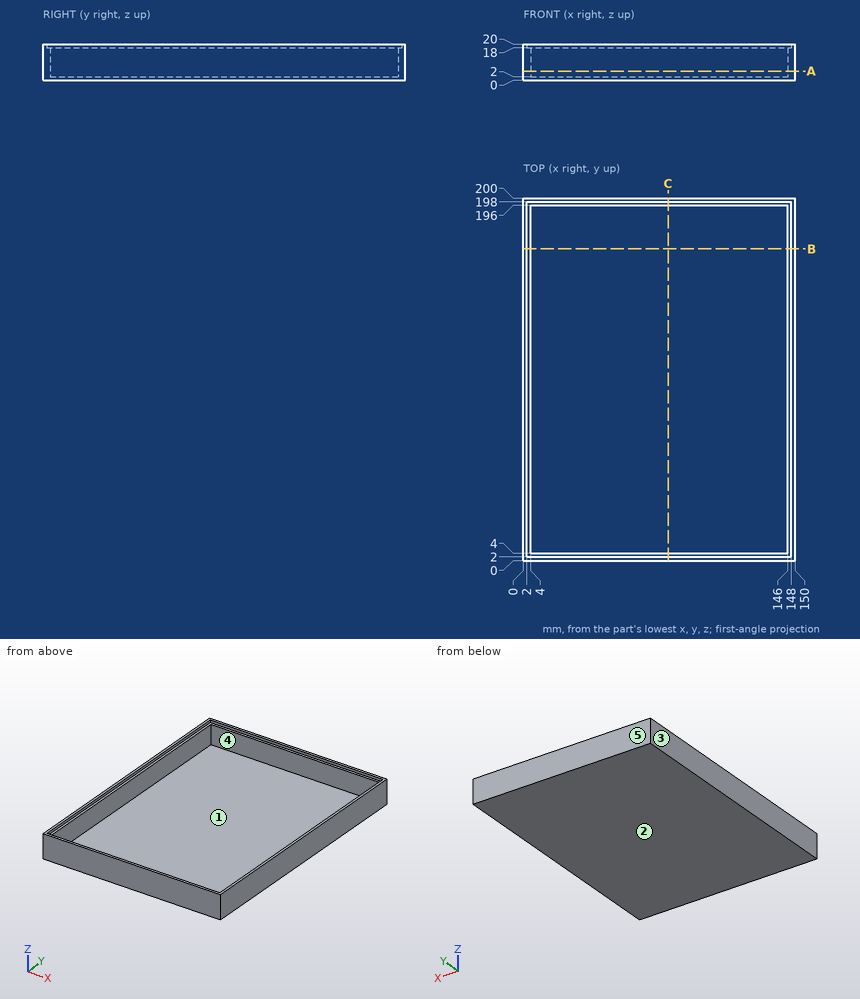
Design review of the part shown in the three views and the two pictorial views. Dimensions are in mm from the part's minimum x, y and z. A direction names the side the tool comes from. Coordinates: 2 decimals unless noted, no trailing zeros. Loops run counter-clockwise (first coordinate to the right, second up) from the corner with the lowest first, then second, coordinate; pieces in that order, holes last. Notation, with made-up numbers: M 18,87 L 36,87 A26 cw 36,105 Z; hole C 40.5,79 d11. An arc over 180 degrees is marked long. One line per question, with ' | ' between items.
(1) We need section B-B (y = 172). Give the boundary of the cut face in (x, z), and give its area (3 significant figures).
Filled in:
outline: M 0,0 L 150,0 L 150,20 L 148,20 L 148,18 L 146,18 L 146,2 L 4,2 L 4,18 L 2,18 L 2,20 L 0,20 Z | area: 436 mm^2
(2) We need section C-C (x = 80). Give the boundary of the cut face in (y, z).
Filled in:
outline: M 0,0 L 200,0 L 200,20 L 198,20 L 198,18 L 196,18 L 196,2 L 4,2 L 4,18 L 2,18 L 2,20 L 0,20 Z
(3) Machinability: for the marked faces 1 and 2, which of the approach directions +Z, -Z, +X, -X, +Y, -Y give a long, thin tool a straight path to every point of the face, cutting with its end or side? Answer none if there is none.
Filled in:
face 1: +Z | face 2: -Z, +X, -X, +Y, -Y
(4) Draft analysis for pull direction X (two halves, no side actions). For the marked faces 3, 4 and 5, state which applies: released by +X, released by -X, zero draft, split by the parting line, or undercut.
Filled in:
face 3: released by -X | face 4: undercut | face 5: zero draft
(5) We need section A-A (z = 5). Give the boundary of the cut face in (x, y).
Filled in:
outline: M 0,0 L 150,0 L 150,200 L 0,200 Z; hole M 4,4 L 146,4 L 146,196 L 4,196 Z
(6) Wall thickness on probe 1 along Y at (x, z) = (31, 17); probe 2 along X at (y, z) = (95, 2.25); probe 3 along X at (y, z) = (124.5, 18.5): over which ranges is each line inside the solid? List them lowest first.
Filled in:
probe 1: y = 0 to 4, 196 to 200 | probe 2: x = 0 to 4, 146 to 150 | probe 3: x = 0 to 2, 148 to 150
(7) For pin 1 Ø4 at (x, z) = (80, 11) entering from -Y, flat-tipped, find the tip position at first contact; note if it passes through.
Filled in:
pin 1: stops at y = 0
